Build history of the part. All positions in model axes, mm. A direction names the side the tool comes from. Round coordinates to 2 decimals unless told otherwise and drop trailing zeros. Write each loop counter-clockwise with the first axis right and the second up, starting at its lowest first coordinate (ties: lowest second). Pieces come first, ordered by that corner, then holes.
1) Pull direction X, two halves, no side cores. Call faces 6 (the flat face through (-1, 3, -3)), 7 (the flat face through (7, 3, -1)), 8 (the flat face through (17, 3, -1)): +X half, -X half, draft (parallel to the pull), parting line (faces both ways), or undercut.
2) Saw through at C-C (y = 5). Write the cut outline in (x, z).
3) Flat gauge pins, fed straight in: pin 1 (2 mm diameter, centred on y = 2, z = 8.5, fed in from +X); pin 2 (3 mm diameter, centred on x = -2, z = 5, fed in from +Y); pin 3 (3 mm diameter, centred on x = -4.5, y = 4, fed in from +Z); pin 4 (2 mm diameter, centred on x = -4.5, y = 4.5, fed in from -Z). Where does each tip first touch, or does it go through?
4) Which spindle directions (+Z, -Z, +X, -X, +Y, -Y) get a long thin tool onto all of the face, cutting with end or side? Do faces 1 (the flat face through (-3, 3, -1)), 2 (the flat face through (14, 2, 5)), 3 (the flat face through (15, 2, 5)), 4 (the flat face through (0, 3, -3)), 5 (the flat face through (15, 3, -3)). Say none if no direction does.
5) Saw through at D-D (x = 6.5). Write the cut outline in (y, z).
6) Saw through at B-B (y = 0.5). State how many separate pieces and enclosed holes the cut face has, plus the area to 3 significant figures.
7) Saw through at A-A (z = 0.5). Write the cut outline in (x, y), plus the area to 3 significant figures.
8) Wall check: probe 1 along X at (y, z) = (3.25, 4); probe 2 along Z at (x, y) = (12.5, 3.25); probe 3 along Y at (x, z) = (19.5, -3). Give the ranges that are in metal, low to high.
from build123d import *

# Parameters (mm, degrees)
BOSS_EXTRUDE5_DEPTH = 1
BOSS_EXTRUDE6_DEPTH = 5
BOSS_EXTRUDE7_DEPTH = 5
BOSS_EXTRUDE8_DEPTH = 5
CUT_EXTRUDE2_DEPTH  = 27.226956509
CUT_EXTRUDE3_DEPTH  = 27.226956509
CUT_EXTRUDE4_DEPTH  = 26.860820726
FILLET1_R           = 1
SKETCH2_10_R        = 1.5
CUT_EXTRUDE5_DEPTH  = 26.372860474
FILLET2_R           = 1
FILLET3_R           = 2


with BuildPart() as part:
    # Sketch2 → Boss-Extrude5 (new body)
    with BuildSketch(Plane(origin=(0, 0, 0), x_dir=(1, 0, 0), z_dir=(0, 1, 0))):
        with BuildLine():
            Line((-2.70717244, 7.535599565), (-1, 5.828427125))
            Line((-1, 5.828427125), (0, 4.828427125))
            Line((0, 4.828427125), (1.393918238, 3.434508886))
            ThreePointArc((1.393918238, 3.434508886), (7, 1.112393789), (12.606081762, 3.434508886))
            Line((12.606081762, 3.434508886), (14, 4.828427125))
            Line((14, 4.828427125), (15, 5.828427125))
            Line((15, 5.828427125), (16.70717244, 7.535599565))
            Line((16.70717244, 7.535599565), (18.70717244, 7.535599565))
            Line((18.70717244, 7.535599565), (20.121386002, 6.121386002))
            Line((20.121386002, 6.121386002), (21.535599565, 4.70717244))
            Line((21.535599565, 4.70717244), (21.535599565, 2.70717244))
            Line((21.535599565, 2.70717244), (19.828427125, 1))
            Line((19.828427125, 1), (18.828427125, 0))
            Line((18.828427125, 0), (17.928932188, -0.899494937))
            ThreePointArc((17.928932188, -0.899494937), (15.761204675, -4.143728425), (15, -7.970562748))
            Line((15, -7.970562748), (15, -12))
            Line((15, -12), (14, -12))
            Line((14, -12), (14, 0))
            Line((14, 0), (0, 0))
            Line((0, 0), (0, -12))
            Line((0, -12), (-1, -12))
            Line((-1, -12), (-1, -7.970562748))
            ThreePointArc((-1, -7.970562748), (-1.761204675, -4.143728425), (-3.928932188, -0.899494937))
            Line((-3.928932188, -0.899494937), (-4.828427125, 0))
            Line((-4.828427125, 0), (-5.828427125, 1))
            Line((-5.828427125, 1), (-7.535599565, 2.70717244))
            Line((-7.535599565, 2.70717244), (-7.535599565, 4.70717244))
            Line((-7.535599565, 4.70717244), (-6.121386002, 6.121386002))
            Line((-6.121386002, 6.121386002), (-4.70717244, 7.535599565))
            Line((-4.70717244, 7.535599565), (-2.70717244, 7.535599565))
        make_face()
    extrude(amount=BOSS_EXTRUDE5_DEPTH)

    # Sketch5 → Boss-Extrude6 (add)
    with BuildSketch(Plane(origin=(0, 1, 0), x_dir=(1, 0, 0), z_dir=(0, 1, 0))):
        Polygon((-4.828427125, 0), (18.828427125, 0), (19.828427125, 1), (-5.828427125, 1), align=None)
    extrude(amount=BOSS_EXTRUDE6_DEPTH)

    # Sketch5<3> → Boss-Extrude7 (add)
    with BuildSketch(Plane(origin=(0, 1, 0), x_dir=(1, 0, 0), z_dir=(0, 1, 0))):
        Polygon((-1, -12), (-1, 5.828427125), (0, 4.828427125), (0, -12), align=None)
    extrude(amount=BOSS_EXTRUDE7_DEPTH)

    # Sketch5<4> → Boss-Extrude8 (add)
    with BuildSketch(Plane(origin=(0, 1, 0), x_dir=(1, 0, 0), z_dir=(0, 1, 0))):
        Polygon((15, -12), (15, 5.828427125), (14, 4.828427125), (14, -12), align=None)
    extrude(amount=BOSS_EXTRUDE8_DEPTH)

    # Sketch6 → Cut-Extrude2 (cut, through all)
    with BuildSketch(Plane.ZY.offset(1)):
        Polygon((12, 1), (0, 6), (12, 6), align=None)
    extrude(amount=-CUT_EXTRUDE2_DEPTH, mode=Mode.SUBTRACT)

    # Sketch7 → Cut-Extrude3 (cut, through all)
    with BuildSketch(Plane.ZY.offset(1)):
        Polygon((-5.828427125, 1), (-1, 6), (-5.828427125, 6), align=None)
    extrude(amount=-CUT_EXTRUDE3_DEPTH, mode=Mode.SUBTRACT)

    # Sketch9 → Cut-Extrude4 (cut, through all)
    with BuildSketch(Plane(origin=(0, 0, -1), x_dir=(-1, 0, 0), z_dir=(0, 0, -1))):
        Polygon((5.828427125, 1), (1, 6), (5.828427125, 6), align=None)
        Polygon((-15, 6), (-19.828427125, 6), (-19.828427125, 1), align=None)
    extrude(amount=-CUT_EXTRUDE4_DEPTH, mode=Mode.SUBTRACT)

    # Fillet1
    fillet1_edges = [part.edges().sort_by_distance(p)[0] for p in [
        (21.535599565, 0.5, -2.70717244),
        (21.535599565, 0.5, -4.70717244),
        (18.70717244, 0.5, -7.535599565),
        (16.70717244, 0.5, -7.535599565),
    ]]
    fillet(fillet1_edges, radius=FILLET1_R)

    # Sketch2<10> → Cut-Extrude5 (cut, through all)
    with BuildSketch(Plane(origin=(0, 0, 0), x_dir=(1, 0, 0), z_dir=(0, 1, 0))):
        with Locations(Location((-4.000065659, 4.000065659, 0), (0, 0, 270))):
            Circle(SKETCH2_10_R)
        with Locations(Location((18.000065659, 4.000065659, 0), (0, 0, 90))):
            Circle(SKETCH2_10_R)
    extrude(amount=CUT_EXTRUDE5_DEPTH, mode=Mode.SUBTRACT)

    # Fillet2
    fillet2_edges = [part.edges().sort_by_distance(p)[0] for p in [
        (-4.70717244, 0.5, -7.535599565),
        (-7.535599565, 0.5, -4.70717244),
        (-7.535599565, 0.5, -2.70717244),
        (-2.70717244, 0.5, -7.535599565),
    ]]
    fillet(fillet2_edges, radius=FILLET2_R)

    # Fillet3
    # the kernel refuses this fillet: 2 mm, written as the material it takes off along each edge
    with BuildSketch(Plane(origin=(16.627933811, -0.685780658, -7.456360936), x_dir=(-0.41774894469873675, -0.8068281343670279, 0.4177489446987422), z_dir=(-0.5705136450630144, 0.5907862232600055, 0.5705136450630186))) as fillet3_piece_1_section:
        with BuildLine():
            CenterArc((FILLET3_R * 0.570690578744, FILLET3_R), FILLET3_R, 210.574008732, 59.425991268)
            Line((-FILLET3_R * 0.290282277773, FILLET3_R * 0.491349097769), (0, 0))
            Line((0, 0), (FILLET3_R * 0.570690578744, 0))
        make_face()
    fillet3_piece_1 = extrude(amount=7.459712243, mode=Mode.PRIVATE)
    fillet3_piece_1 = split(fillet3_piece_1, bisect_by=Plane(origin=(16.627933811, 1, -7.456360936), z_dir=(0, 1, 0)), keep=Keep.TOP, mode=Mode.PRIVATE)
    add(fillet3_piece_1, mode=Mode.SUBTRACT)
    with BuildSketch(Plane(origin=(1.627933811, 3.721314564, -3.200493313), x_dir=(0.41774894469873974, -0.8068281343670296, 0.41774894469873625), z_dir=(-0.5705136450630193, -0.5907862232600034, -0.5705136450630159))) as fillet3_piece_2_section:
        with BuildLine():
            CenterArc((FILLET3_R * 0.570690578744, FILLET3_R), FILLET3_R, 210.574008732, 59.425991268)
            Line((-FILLET3_R * 0.290282277773, FILLET3_R * 0.491349097769), (0, 0))
            Line((0, 0), (FILLET3_R * 0.570690578744, 0))
        make_face()
    fillet3_piece_2 = extrude(amount=7.459712243, mode=Mode.PRIVATE)
    fillet3_piece_2 = split(fillet3_piece_2, bisect_by=Plane(origin=(1.627933811, 1, -3.200493313), z_dir=(0, 1, 0)), keep=Keep.TOP, mode=Mode.PRIVATE)
    add(fillet3_piece_2, mode=Mode.SUBTRACT)
    with BuildSketch(Plane(origin=(-3.200493313, 3.721314564, 1.627933811), x_dir=(0.417748944698757, -0.8068281343670092, 0.4177489446987582), z_dir=(-0.570513645063002, -0.5907862232600312, -0.5705136450630045))) as fillet3_piece_3_section:
        with BuildLine():
            CenterArc((FILLET3_R * 0.570690578744, -FILLET3_R), FILLET3_R, 90, 59.425991268)
            Line((-FILLET3_R * 0.290282277773, -FILLET3_R * 0.491349097769), (0, 0))
            Line((0, 0), (FILLET3_R * 0.570690578744, 0))
        make_face()
    fillet3_piece_3 = extrude(amount=7.459712243, mode=Mode.PRIVATE)
    fillet3_piece_3 = split(fillet3_piece_3, bisect_by=Plane(origin=(-3.200493313, 1, 1.627933811), z_dir=(0, 1, 0)), keep=Keep.TOP, mode=Mode.PRIVATE)
    add(fillet3_piece_3, mode=Mode.SUBTRACT)
    with BuildSketch(Plane(origin=(17.200493313, 3.721314564, 1.627933811), x_dir=(-0.4177489446987597, -0.8068281343670061, 0.41774894469876167), z_dir=(0.5705136450629996, -0.5907862232600355, -0.5705136450630022))) as fillet3_piece_4_section:
        with BuildLine():
            CenterArc((FILLET3_R * 0.570690578744, FILLET3_R), FILLET3_R, 210.574008732, 59.425991268)
            Line((-FILLET3_R * 0.290282277773, FILLET3_R * 0.491349097769), (0, 0))
            Line((0, 0), (FILLET3_R * 0.570690578744, 0))
        make_face()
    fillet3_piece_4 = extrude(amount=7.459712243, mode=Mode.PRIVATE)
    fillet3_piece_4 = split(fillet3_piece_4, bisect_by=Plane(origin=(17.200493313, 1, 1.627933811), z_dir=(0, 1, 0)), keep=Keep.TOP, mode=Mode.PRIVATE)
    add(fillet3_piece_4, mode=Mode.SUBTRACT)
    with BuildSketch(Plane(origin=(10.748288019, 1, 12), x_dir=(0, -1, 0), z_dir=(1, 0, 0)), Plane(origin=(-4.251711981, 1, 12), x_dir=(0, -1, 0), z_dir=(1, 0, 0))) as fillet3_piece_5:
        with BuildLine():
            CenterArc((1.345890464, 1.969862885), FILLET3_R, 202.619864948, 57.421029607)
            Line((-0.500263382, 1.200632116), (0, 0))
            Line((0, 0), (1, 0))
        make_face()
    extrude(amount=7.503423962, mode=Mode.SUBTRACT)


solid = part.part
Evaluation:
1. face 6: -X half
1. face 7: undercut
1. face 8: draft
2. outline: (-1.97, -1) - (-1, -1) - (-1, -1.97) - (0, -1.97) - (0, -1) - (14, -1) - (14, -1.97) - (15, -1.97) - (15, -1) - (15.97, -1) - (15.97, 0) - (15, 0) - (15, 2.4) - (14, 2.4) - (14, 0) - (0, 0) - (0, 2.4) - (-1, 2.4) - (-1, 0) - (-1.97, 0) - close
3. pin 1: stops at x = 15
3. pin 2: stops at y = 4.38
3. pin 3: stops at z = 0
3. pin 4: passes through
4. face 1: -Z, -X, +Y
4. face 2: +Z, +Y, -Y
4. face 3: +Z, +X, +Y
4. face 4: -Z, +Y
4. face 5: -Z, +X, +Y
5. outline: (0, -1.13) - (1, -1.13) - (1, -1) - (6, -1) - (6, 0) - (0, 0) - close
6. separate pieces: 1
6. enclosed holes: 2
6. area: 151 mm2
7. outline: (-4.33, 0) - (0, 0) - (0, 5.79) - (-1, 5.79) - (-1, 1) - (-4.33, 1) - close; (14, 0) - (18.33, 0) - (18.33, 1) - (15, 1) - (15, 5.79) - (14, 5.79) - close
7. area: 18.2 mm2
8. probe 1: x = -1 to 0, 14 to 15
8. probe 2: z = -1 to 0
8. probe 3: y = 0 to 1
